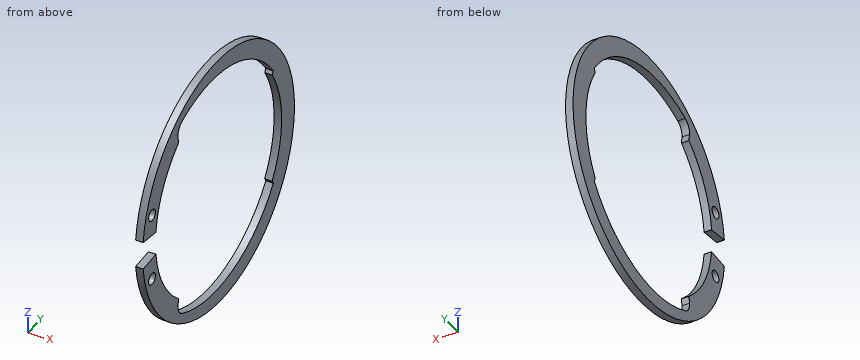
Autodesk Inventor part; units mm, degrees
ref_plane "YZ Plane" through (0, 0, 0) normal (1, 0, 0) x (0, 1, 0)
ref_plane "XZ Plane" through (0, 0, 0) normal (0, 1, 0) x (-1, 0, 0)
ref_plane "XY Plane" through (0, 0, 0) normal (0, 0, 1) x (1, 0, 0)
sketch "Sketch1" plane through (0, 0, 0) normal (0, 0, 1) x (1, 0, 0)
  line L0 (0, 0) -> (-75.2784, 0)
  line L1 (0, 28.5) -> (-2, 28.5)
  line L2 (-2, 28.5) -> (-2, 34.3)
  line L3 (-2, 34.3) -> (0, 34.3)
  line L4 (0, 34.3) -> (0, 28.5)
  point P0 (0, 0)
  dimension "d0" = 2
  dimension "d1" = 57
  dimension "d2" = 68.6
revolve "Revolution1" add sketch "Sketch1" angle 360 about axis through (0, 0, 0) along (-1, 0, 0)
sketch "Sketch2" plane through (0, 0, 0) normal (1, 0, 0) x (0, 0, -1)
  circle A0 centre (0, 0) radius 28.5
  line L0 (0, 0) -> (15, 24.2332) construction
  line L1 (0, 0) -> (-15, 24.2332) construction
  line L2 (0, 0) -> (3.1, -28.3309) construction
  line L3 (0, 0) -> (-3.1, -28.3309) construction
  circle A1 centre (0, 0) radius 34.3
  line L4 (3.1, -28.3309) -> (3.7309, -34.0965)
  line L5 (-3.1, -28.3309) -> (-3.7309, -34.0965)
  line L6 (15, 24.2332) -> (15.8503, 24.7596)
  line L7 (-15, 24.2332) -> (-15.8503, 24.7596)
  line L8 (0, 0) -> (22, -18.1177) construction
  line L9 (0, 0) -> (-22, -18.1177) construction
  circle A2 centre (0, 0) radius 31.8 construction
  line L10 (-22, -18.1177) -> (-23.8497, -18.3201)
  line L11 (22, -18.1177) -> (23.8497, -18.3201)
  arc A3 (-27.1979, -16.4377) -> (-23.8497, -18.3201) centre (-24.2087, -15.0396) ccw
  arc A4 (23.8497, -18.3201) -> (27.1979, -16.4377) centre (24.2087, -15.0396) ccw
  arc A5 (-15.8503, 24.7596) -> (-27.1979, -16.4377) centre (2.6227, -2.4902) ccw
  arc A6 (27.1979, -16.4377) -> (15.8503, 24.7596) centre (-2.6227, -2.4902) ccw
  circle A7 centre (0, 0) radius 31.4 construction
  line L12 (3.4154, -31.2137) -> (18.4181, -29.5721) construction
  circle A8 centre (9, -30.0826) radius 1.55
  circle A9 centre (-9, -30.0826) radius 1.55
  dimension "d4" = 30
  dimension "d5" = 6.2
  dimension "d6" = 1
  dimension "d7" = 44
  dimension "d8" = 2.5
  dimension "d9" = 32.9211
  dimension "d10" = 3.1
  dimension "d11" = 18
extrude "Extrusion1" cut sketch "Sketch2" against normal through all contours A0 L6 A6 A4 L11 | A0 L10 A3 A5 L7 | L4 A1 L5 A0 | A8 | A9
properties part number "3136 7009 59"
Design review of the part built by this model. Coordinates are the model's own, in mm. Round coordinates to 2 decimals unless told otherwise and drop trailing zeros. Loops run counter-clockwise (first coordinate to the right, second up) from the corner with the lowest first, then second, coordinate; pieces in that order, holes last. Notation, with made-up numbers: (52, 77) -> (88, 77) arc R31 ccw to (88, 106) -> close; hole circle Ø3 at (-31.75, -5). An arc over 180 degrees is marked (long way). Use one line per item in the form item = value. Start each with the question number.
Q1. We need section D-D on z = 0. Give the boundary of the cut face in (x, y), then the cut area to 3 significant figures.
Q2. We need section B-B on y = -4. Give the boundary of the cut face in (x, z).
Q3. We need section A-A on z = -12.5. Give the boundary of the cut face in (x, y).
Q4. Wall thickness on line 1 along Y through (x, z) = (-1.8, 5); line 2 along Y through (x, z) = (-0.2, -15); line 3 along Y through (x, z) = (-0.5, 9): over which ranges is each line inside the solid? List them lowest first. Write a range as [from, to].
Q5. We need section C-C on x = -1. Give the boundary of the cut face in (y, z), then the cut area to 3 significant figures.
Q6. For pin 1 Ø1.9 at (y, z) = (-30.08, -9) entering from -X, flat-tipped, find the tip position at first contact; note if it passes through.
Calculated:
q1.outline = (-2, 28.5) -> (0, 28.5) -> (0, 34.3) -> (-2, 34.3) -> close
q1.area = 11.6 mm²
q2.outline = (-2, -34.07) -> (0, -34.07) -> (0, -30.26) -> (-2, -30.26) -> close; (-2, 30.26) -> (0, 30.26) -> (0, 34.07) -> (-2, 34.07) -> close
q3.outline = (-2, -31.94) -> (0, -31.94) -> (0, -25.61) -> (-2, -25.61) -> close; (-2, 25.61) -> (0, 25.61) -> (0, 31.94) -> (-2, 31.94) -> close
q4.line_1 = [-33.93, -28.06], [28.06, 33.93]
q4.line_2 = [-30.85, -24.23], [24.23, 30.85]
q4.line_3 = [-33.1, -31.63], [-28.53, -27.04], [27.04, 33.1]
q5.outline = (-34.1, -3.73) arc R34.3 ccw (long way) to (-34.1, 3.73) -> (-28.33, 3.1) arc R28.5 cw to (-18.12, 22) -> (-18.32, 23.85) arc R3.3 cw to (-16.44, 27.2) arc R32.92 cw to (24.76, 15.85) -> (24.23, 15) arc R28.5 cw to (24.23, -15) -> (24.76, -15.85) arc R32.92 cw to (-16.44, -27.2) arc R3.3 cw to (-18.32, -23.85) -> (-18.12, -22) arc R28.5 cw to (-28.33, -3.1) -> close; hole circle Ø3.1 at (-30.08, -9); hole circle Ø3.1 at (-30.08, 9)
q5.area = 929 mm²
q6.pin_1 = through
